```python
from build123d import *

# Parameters (mm, degrees)
EXTRUDE_1_DEPTH      = 2.5
EXTRUDE_2_DEPTH      = 10.45
EXTRUDE_2_DEPTH_BACK = 10.45


with BuildPart() as part:
    # 스케치2 → 보스-돌출1 (new body)
    with BuildSketch(Plane(origin=(0, 0, 0), x_dir=(1, 0, 0), z_dir=(0, 1, 0))):
        Polygon((-10.45, 12.5), (10.45, 12.5), (10.45, 8.49), (12.309935206, 8.49), (12.309935206, 3.49), (10.45, 3.49), (10.45, -3.49), (12.309935206, -3.49), (12.309935206, -8.49), (10.45, -8.49), (10.45, -12.5), (-10.45, -12.5), (-10.45, -8.49), (-12.309935206, -8.49), (-12.309935206, -3.49), (-10.45, -3.49), (-10.45, 3.49), (-12.309935206, 3.49), (-12.309935206, 8.49), (-10.45, 8.49), align=None)
    extrude(amount=EXTRUDE_1_DEPTH)

    # 스케치3 → 보스-돌출2 (add, two sides: drawn at the far end of the back side and taken through both)
    with BuildSketch(Plane(origin=(0, 0, 0), x_dir=(0, 0, -1), z_dir=(1, 0, 0)).offset(-EXTRUDE_2_DEPTH_BACK)):
        Polygon((0, 0), (12.5, 0), (15.446494384, 0.816274423), (17.628816823, 2.372016775), (18.685999924, 3.881830714), (22.088144039, 10.103695427), (19.588144039, 10.103695427), (15.289438896, 3.964508245), (14.076540474, 3.115227628), (12.22303717, 2.5), (-12.347890055, 2.5), (-12.22303717, 2.5), (-14.076540474, 3.115227628), (-15.289438896, 3.964508245), (-19.588144039, 10.103695427), (-22.088144039, 10.103695427), (-18.685999924, 3.881830714), (-17.628816823, 2.372016775), (-15.446494384, 0.816274423), (-12.5, 0), align=None)
    extrude(amount=EXTRUDE_2_DEPTH + EXTRUDE_2_DEPTH_BACK)


solid = part.part
```
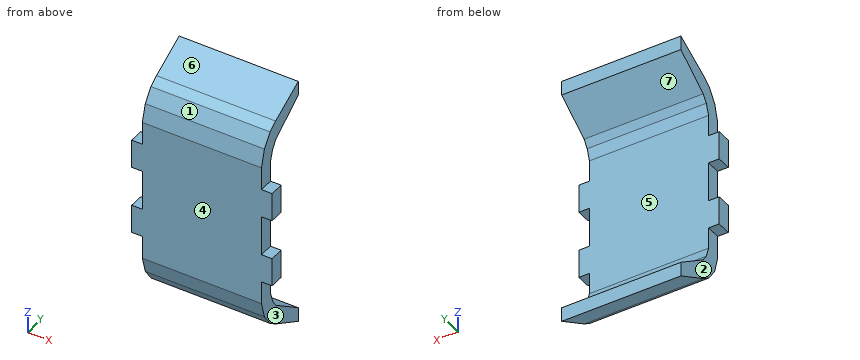
The model under review builds one solid part; all positions refer to its coordinate system, in mm. Face numbers are marked on the shaded views. A direction names the side the tool comes from. Give positions to 0.01 mm unless a question says otherwise; leave off trailing zeros. Write each loop counter-clockwise with the first axis right and the second up, starting at its lowest first coordinate (ties: lowest second). Pieces come first, ordered by that corner, then holes. Notation, with made-up numbers: (-18.5, 83) - (37.5, 83) arc R21 cw to (37.5, 106) - close; hole circle Ø4 at (14, 57.5). An arc over 180 degrees is marked (long way). Answer in a Markdown table with one row per item. Add a question column.
1. We need section D-D on z = 13. Write out the cut boundary in (x, y).
2. Draft analysis for pull direction Z (two halves, no side actions). For the marked faces 4, 5, 6 and 7, state which applies: +Z half, -Z half, draft (parallel to the pull), parting line (faces both ways), or undercut.
3. Insertion check: P1, Ø1, axis at x = -9, y = 6.5, coming from the +Z side; P2, Ø3, axis at y = 1.5, z = -0.5, coming from the +X side; P3, Ø0.6, axis at x = 11, y = 1.5, coming from the -Z side. Each pin has a flat end and moves straight along its axis. Give the tip position at first contact, or say it passes through.
4. Tool access review of the marked faces 1, 2 and 3: name each direction out of +Z, -Z, +X, -X, +Y, -Y from which nothing blocks a thin tool from reaching the whole face with its end or side.
5. We need section C-C on z = -4. Write out the cut boundary in (x, y), then the cut area to 3 significant figures.
6. We need section B-B on x = -8. Write out the cut boundary in (y, z), then the cut area to 3 significant figures.
7. Wall thickness on line 1 along Z through (x, y) = (-10.5, 0.5); line 2 along Y through (x, z) = (8.5, -7); line 3 along Z through (x, y) = (-9.5, 7.5): over which ranges is each line inside the solid? List them lowest first. Write a range as [from, to].
8. We need section A-A on y = 6.75. Write out the cut boundary in (x, z), then the cut area to 3 significant figures.
Ans:
| question | item | result |
|---|---|---|
| 1 | outline | (-10.45, 0.14) - (10.45, 0.14) - (10.45, 2.76) - (-10.45, 2.76) - close |
| 2 | face 4 | draft |
| 2 | face 5 | undercut |
| 2 | face 6 | +Z half |
| 2 | face 7 | undercut |
| 3 | P1 | stops at z = 20.39 |
| 3 | P2 | stops at x = 10.45 |
| 3 | P3 | stops at z = -8.49 |
| 4 | face 1 | +Z, +X, -X, -Y |
| 4 | face 2 | -Z, -X, +Y, -Y |
| 4 | face 3 | -Z, +X, +Y, -Y |
| 5 | outline | (-12.31, 0) - (12.31, 0) - (12.31, 2.5) - (-12.31, 2.5) - close |
| 5 | area | 61.5 mm^2 |
| 6 | outline | (0, -12.5) - (0.82, -15.45) - (2.37, -17.63) - (3.88, -18.69) - (10.1, -22.09) - (10.1, -19.59) - (3.96, -15.29) - (3.12, -14.08) - (2.5, -12.22) - (2.5, 12.22) - (3.12, 14.08) - (3.96, 15.29) - (10.1, 19.59) - (10.1, 22.09) - (3.88, 18.69) - (2.37, 17.63) - (0.82, 15.45) - (0, 12.5) - close |
| 6 | area | 128 mm^2 |
| 7 | line 1 | z = [-8.49, -3.49], [3.49, 8.49] |
| 7 | line 2 | y = [0, 2.5] |
| 7 | line 3 | z = [-20.66, -17.77], [17.77, 20.66] |
| 8 | outline | (-10.45, -20.25) - (10.45, -20.25) - (10.45, -17.24) - (-10.45, -17.24) - close; (-10.45, 17.24) - (10.45, 17.24) - (10.45, 20.25) - (-10.45, 20.25) - close |
| 8 | area | 126 mm^2 |
